Here's how the part is built. I have some questions about the finished solid (model axes, mm). A direction names the side the tool comes from. Give positions to 0.01 mm unless a question says otherwise; leave off trailing zeros. Order: outer loops, then holes, each group sorted by start corner. A loop starts at its lowest first (then second) coordinate and runs counter-clockwise, first axis right, second up.
from build123d import *

# Parameters (mm, degrees)
BOSS_EXTRUDE1_DEPTH            = 4
HOLE1_D                        = 6.6
HOLE1_CBORE_D                  = 11.5
HOLE1_CBORE_DEPTH              = 2
CUT_EXTRUDE3_DEPTH             = 110.27488275
CBORE_FOR_M3_SHCS1_D           = 3.4
CBORE_FOR_M3_SHCS1_CBORE_D     = 6.5
CBORE_FOR_M3_SHCS1_CBORE_DEPTH = 3
FILLET4_R                      = 5
FILLET3_R                      = 2


with BuildPart() as part:
    # Sketch2 → Boss-Extrude1 (new body)
    with BuildSketch(Plane(origin=(0, 0, 0), x_dir=(1, 0, 0), z_dir=(0, 1, 0))):
        with BuildLine():
            Line((-30, -45), (-7.721394619, -18.449391999))
            ThreePointArc((-7.721394619, -18.449391999), (0, -20), (7.721394619, -18.449391999))
            Line((7.721394619, -18.449391999), (30, -45))
            Line((30, -45), (30, -105))
            Line((30, -105), (-30, -105))
            Line((-30, -105), (-30, -45))
        make_face()
    extrude(amount=BOSS_EXTRUDE1_DEPTH)

    # Hole1 (through all)
    with Locations(Plane(origin=(0, 4, 0), x_dir=(1, 0, 0), z_dir=(0, 1, 0))):
        with Locations((-25, -100), (25, -100), (0, -25)):
            CounterBoreHole(HOLE1_D / 2, HOLE1_CBORE_D / 2, HOLE1_CBORE_DEPTH)

    # Sketch5 → Cut-Extrude3 (cut, through all)
    with BuildSketch(Plane(origin=(0, 4, 0), x_dir=(1, 0, 0), z_dir=(0, 1, 0))):
        with BuildLine():
            Line((-30, -102.839454173), (-30, -105))
            Line((-30, -105), (-27.839454173, -105))
            ThreePointArc((-27.839454173, -105), (-29.065863992, -104.065863992), (-30, -102.839454173))
        make_face()
        with BuildLine():
            Line((30, -105), (27.839454173, -105))
            ThreePointArc((27.839454173, -105), (29.065863992, -104.065863992), (30, -102.839454173))
            Line((30, -102.839454173), (30, -105))
        make_face()
    extrude(amount=-CUT_EXTRUDE3_DEPTH, mode=Mode.SUBTRACT)

    # CBORE for M3 SHCS1 (through all)
    with Locations(Plane(origin=(0, 0, 0), x_dir=(-1, 0, 0), z_dir=(0, -1, 0))):
        with Locations((-15.5, -56.9), (15.5, -56.9), (15.5, -87.9), (-15.5, -87.9)):
            CounterBoreHole(CBORE_FOR_M3_SHCS1_D / 2, CBORE_FOR_M3_SHCS1_CBORE_D / 2, CBORE_FOR_M3_SHCS1_CBORE_DEPTH)

    # Fillet4
    fillet4_edges = [part.edges().sort_by_distance(p)[0] for p in [
        (-30, 2, 45),
        (-7.721394619, 2, 18.449391999),
        (7.721394619, 2, 18.449391999),
        (30, 2, 45),
    ]]
    fillet(fillet4_edges, radius=FILLET4_R)

    # Fillet3
    fillet3_edges = [part.edges().sort_by_distance(p)[0] for p in [
        (30, 4, 71.990198499),
        (0, 4, 105),
        (-30, 4, 71.990198499),
        (-19.362432028, 4, 32.322640153),
        (-29.698463104, 4, 45.109750455),
        (-3.699480023, 4, 19.654868292),
        (-7.607899613, 4, 19.497501458),
        (29.698463104, 4, 45.109750455),
        (19.362432028, 4, 32.322640153),
        (7.607899613, 4, 19.497501458),
        (3.699480023, 4, 19.654868292),
    ]]
    fillet(fillet3_edges, radius=FILLET3_R)


solid = part.part
Q1. If we section it at B-B on z = 87.9: List the corners of the cut face in (x, y) for me.
Filled sheet:
outline: (-30, 0) - (-18.75, 0) - (-18.75, 3) - (-17.2, 3) - (-17.2, 4) - (-28, 4) arc R2 ccw to (-30, 2) - close; (-13.8, 3) - (-12.25, 3) - (-12.25, 0) - (12.25, 0) - (12.25, 3) - (13.8, 3) - (13.8, 4) - (-13.8, 4) - close; (17.2, 3) - (18.75, 3) - (18.75, 0) - (30, 0) - (30, 2) arc R2 ccw to (28, 4) - (17.2, 4) - close
Q2. If we section it at C-C on x = -15.5: Give the number of separate pieces and of enclosed holes in the cut face, plus the area to 3 significant figures.
Filled sheet:
separate pieces: 3
enclosed holes: 0
area: 261 mm2
Q3. I'm going to push flat-ended pins straight in: P1, Ø4, axis at x = 25, z = 100, coming from the -Y side; P2, Ø10.5, axis at x = 0, z = 25, coming from the +Y side; P3, Ø5, axis at x = -15, z = 57, coming from the -Y side; P4, Ø1, axis at x = 9, y = 2.5, coming from the -Z side. Where does each tip first touch, or does it pass through?
Filled sheet:
P1: passes through
P2: stops at y = 2
P3: stops at y = 3
P4: stops at z = 19.93
Q4. If we section it at A-A on z = 100: List the corners of the cut face in (x, y) for me.
Filled sheet:
outline: (-30, 0) - (-28.3, 0) - (-28.3, 2) - (-30, 2) - close; (-21.7, 0) - (21.7, 0) - (21.7, 2) - (19.25, 2) - (19.25, 4) - (-19.25, 4) - (-19.25, 2) - (-21.7, 2) - close; (28.3, 0) - (30, 0) - (30, 2) - (28.3, 2) - close
Q5. I need wall thicknesses on L1, parallel to X at y = 1.5, z = 100; L2, parallel to Z at x = 15.5, y = 1.65; L3, parallel to X at y = 3.6, z = 55.5. Which ranges of each line are inside material? Lowest first, please.
Filled sheet:
L1: x = -30 to -28.3, -21.7 to 21.7, 28.3 to 30
L2: z = 27.72 to 53.65, 60.15 to 84.65, 91.15 to 105
L3: x = -29.2 to -16.46, -14.54 to 14.54, 16.46 to 29.2
Q6. For faces 1 (the face through (21.04, 3.01, 95.83)), 2 (the face through (0, 0, 62)), 3 (the face through (-15.077, 1.479, 84.678)), which set-ups out of +Z, -Z, +X, -X, +Y, -Y let a thin tool reach every point of the face, with its end or its side?
Filled sheet:
face 1: +Y
face 2: +Z, -Z, +X, -X, -Y
face 3: -Y
